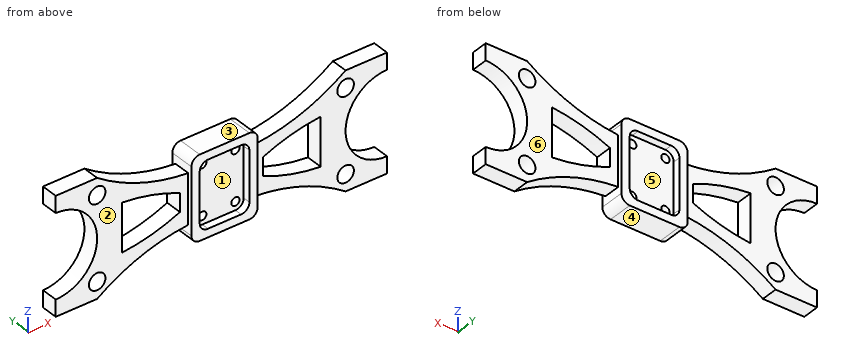
from build123d import *

# Parameters (mm, degrees)
SKETCH1_R             = 5
BOSS_EXTRUDE1_DEPTH   = 5
BOSS_EXTRUDE1_2_DEPTH = 5
SKETCH1_3_R           = 2.5
BOSS_EXTRUDE2_DEPTH   = 3
BOSS_EXTRUDE3_DEPTH   = 7.5


with BuildPart() as part:
    # Sketch1 → Boss-Extrude1 (new, symmetric)
    with BuildSketch(Plane(origin=(0, 0, 0), x_dir=(1, 0, 0), z_dir=(0, 1, 0))):
        with BuildLine():
            ThreePointArc((-75, -35), (-48.85448144, -21.27517604), (-20, -15))
            Line((-20, -15), (-20, 15))
            ThreePointArc((-20, 15), (-48.85448144, 21.27517604), (-75, 35))
            Line((-75, 35), (-100, 35))
            Line((-100, 35), (-100, 25))
            ThreePointArc((-100, 25), (-75, 0), (-100, -25))
            Line((-100, -25), (-100, -35))
            Line((-100, -35), (-75, -35))
        make_face()
        with Locations(Location((-75, -25, 0), (0, 0, 270))):
            Circle(SKETCH1_R, mode=Mode.SUBTRACT)
        with BuildLine():
            Line((-60, -14.5), (-60, 14.5))
            ThreePointArc((-60, 14.5), (-42.12787297, 11.447160671), (-25, 5.5))
            Line((-25, 5.5), (-25, -5.5))
            ThreePointArc((-25, -5.5), (-42.12787297, -11.447160671), (-60, -14.5))
        make_face(mode=Mode.SUBTRACT)
        with Locations(Location((-75, 25, 0), (0, 0, 270))):
            Circle(SKETCH1_R, mode=Mode.SUBTRACT)
    extrude(amount=BOSS_EXTRUDE1_DEPTH, both=True)



with BuildPart() as body_2:
    # Sketch1 → Boss-Extrude1 2 (new, symmetric)
    with BuildSketch(Plane(origin=(0, 0, 0), x_dir=(1, 0, 0), z_dir=(0, 1, 0))):
        with BuildLine():
            Line((20, 15), (20, -15))
            ThreePointArc((20, -15), (48.85448144, -21.27517604), (75, -35))
            Line((75, -35), (100, -35))
            Line((100, -35), (100, -25))
            ThreePointArc((100, -25), (75, 0), (100, 25))
            Line((100, 25), (100, 35))
            Line((100, 35), (75, 35))
            ThreePointArc((75, 35), (48.85448144, 21.27517604), (20, 15))
        make_face()
        with Locations(Location((75, -25, 0), (0, 0, 270))):
            Circle(SKETCH1_R, mode=Mode.SUBTRACT)
        with BuildLine():
            ThreePointArc((60, -14.5), (42.12787297, -11.447160671), (25, -5.5))
            Line((25, -5.5), (25, 5.5))
            ThreePointArc((25, 5.5), (42.12787297, 11.447160671), (60, 14.5))
            Line((60, 14.5), (60, -14.5))
        make_face(mode=Mode.SUBTRACT)
        with Locations(Location((75, 25, 0), (0, 0, 270))):
            Circle(SKETCH1_R, mode=Mode.SUBTRACT)
    extrude(amount=BOSS_EXTRUDE1_2_DEPTH, both=True)


with BuildPart() as body_3:
    # Sketch1<3> → Boss-Extrude2 (new, symmetric)
    with BuildSketch(Plane(origin=(0, 0, 0), x_dir=(1, 0, 0), z_dir=(0, 1, 0))):
        with BuildLine():
            Line((15, 15), (15, -15))
            ThreePointArc((15, -15), (13.535533906, -18.535533906), (10, -20))
            Line((10, -20), (-10, -20))
            ThreePointArc((-10, -20), (-13.535533906, -18.535533906), (-15, -15))
            Line((-15, -15), (-15, 15))
            ThreePointArc((-15, 15), (-13.535533906, 18.535533906), (-10, 20))
            Line((-10, 20), (10, 20))
            ThreePointArc((10, 20), (13.535533906, 18.535533906), (15, 15))
        make_face()
        with Locations(Location((10, 15, 0), (0, 0, 270))):
            Circle(SKETCH1_3_R, mode=Mode.SUBTRACT)
        with Locations(Location((-10, 15, 0), (0, 0, 270))):
            Circle(SKETCH1_3_R, mode=Mode.SUBTRACT)
        with Locations(Location((-10, -15, 0), (0, 0, 270))):
            Circle(SKETCH1_3_R, mode=Mode.SUBTRACT)
        with Locations(Location((10, -15, 0), (0, 0, 270))):
            Circle(SKETCH1_3_R, mode=Mode.SUBTRACT)
    extrude(amount=BOSS_EXTRUDE2_DEPTH, both=True)


with BuildPart() as part_1:
    add(part.part)

    add(body_2.part)  # Boss-Extrude3 merges body 2

    add(body_3.part)  # Boss-Extrude3 merges body 3
    # Sketch1<4> → Boss-Extrude3 (add, symmetric)
    with BuildSketch(Plane(origin=(0, 0, 0), x_dir=(1, 0, 0), z_dir=(0, 1, 0))):
        with BuildLine():
            ThreePointArc((-15, -25), (-18.535533906, -23.535533906), (-20, -20))
            Line((-20, -20), (-20, 20))
            ThreePointArc((-20, 20), (-18.535533906, 23.535533906), (-15, 25))
            Line((-15, 25), (15, 25))
            ThreePointArc((15, 25), (18.535533906, 23.535533906), (20, 20))
            Line((20, 20), (20, -20))
            ThreePointArc((20, -20), (18.535533906, -23.535533906), (15, -25))
            Line((15, -25), (-15, -25))
        make_face()
        with BuildLine():
            ThreePointArc((15, 15), (13.535533906, 18.535533906), (10, 20))
            Line((10, 20), (-10, 20))
            ThreePointArc((-10, 20), (-13.535533906, 18.535533906), (-15, 15))
            Line((-15, 15), (-15, -15))
            ThreePointArc((-15, -15), (-13.535533906, -18.535533906), (-10, -20))
            Line((-10, -20), (10, -20))
            ThreePointArc((10, -20), (13.535533906, -18.535533906), (15, -15))
            Line((15, -15), (15, 15))
        make_face(mode=Mode.SUBTRACT)
    extrude(amount=BOSS_EXTRUDE3_DEPTH, both=True)


solid = part_1.part
Could you check a few things on this model? Use its own coordinates, in mm. Face numbers are marked on the shaded views. A direction names the side the tool comes from. Give positions to 0.01 mm unless a question says otherwise; leave off trailing zeros. Loops run counter-clockwise (first coordinate to the right, second up) from the corner with the lowest first, then second, coordinate; pieces in that order, holes last. Notation, with made-up numbers: (8.25, 11.5) -> (21.25, 11.5) arc R30 cw to (21.25, 43.5) -> close; hole circle Ø3 at (17.25, 60). An arc over 180 degrees is marked (long way). Answer as CSV lines item,"result". Start each with the question number.
(1) If we section it at A-A on x = -86.5: Write out the boundary of the cut face in (y, z), then the cut area to 3 significant figures.
(2) If we section it at B-B on z = 2: Write out the boundary of the cut face in (x, y).
(3) I need wall thicknesses on probe 1 along X at (y, z) = (-2, -1); probe 2 along Z at (x, y) = (-9, -5.5); probe 3 along Y at (x, z) = (-89, 24.5). Which ranges of each line are inside material? Lowest first, please.
(4) Which directions (+Z, -Z, +X, -X, +Y, -Y) give clear straight access to the entire face, cutting with the end or side of a thin tool? Please do the marked faces 1, 2 and 3.
(5) If we section it at D-D on x = -2: Write out the boundary of the cut face in (y, z), then the cut area to 3 significant figures.
(6) I'm going to push flat-ended pins straight in: pin 1 Ø24 at (x, z) = (-2, -4) entering from +Y; pin 2 Ø9 at (x, z) = (75, 25) entering from -Y; pin 3 Ø5 at (y, z) = (-5, -0.5) entering from +X; pin 4 Ø3.5 at (x, y) = (1.5, 5.5) entering from -Z. Where does each tip first touch, or does it pass through?
(7) If we section it at C-C on y = 1: Count the separate pieces of the cut face and the enclosed holes in it, then the cut area to 3 significant figures.
(8) We'd pull the mould along Z, two halves only. Please class the marked faces 4, 5 and 6: released by +Z, released by -Z, zero draft, split by the parting line, or undercut.
Computed:
1,outline,"(-5, -35) -> (5, -35) -> (5, -21.04) -> (-5, -21.04) -> close; (-5, 21.04) -> (5, 21.04) -> (5, 35) -> (-5, 35) -> close"
1,area,"279 mm2"
2,outline,"(-75.08, -5) -> (-60, -5) -> (-60, 5) -> (-75.08, 5) -> close; (-25, -5) -> (-20, -5) -> (-20, -7.5) -> (-15, -7.5) -> (-15, -3) -> (15, -3) -> (15, -7.5) -> (20, -7.5) -> (20, -5) -> (25, -5) -> (25, 5) -> (20, 5) -> (20, 7.5) -> (15, 7.5) -> (15, 3) -> (-15, 3) -> (-15, 7.5) -> (-20, 7.5) -> (-20, 5) -> (-25, 5) -> close; (60, -5) -> (75.08, -5) -> (75.08, 5) -> (60, 5) -> close"
3,probe 1,"x = -75.02 to -60, -25 to 25, 60 to 75.02"
3,probe 2,"z = -25 to -20, 20 to 25"
3,probe 3,"y = -5 to 5"
4,face 1,"-Y"
4,face 2,"+Z, -Z, -X, -Y"
4,face 3,"+Z, +Y, -Y"
5,outline,"(-7.5, -25) -> (7.5, -25) -> (7.5, -20) -> (3, -20) -> (3, 20) -> (7.5, 20) -> (7.5, 25) -> (-7.5, 25) -> (-7.5, 20) -> (-3, 20) -> (-3, -20) -> (-7.5, -20) -> close"
5,area,"390 mm2"
6,pin 1,"stops at y = 3"
6,pin 2,"passes through"
6,pin 3,"stops at x = 75.18"
6,pin 4,"stops at z = -25"
7,separate pieces,"1"
7,enclosed holes,"10"
7,area,"6,460 mm2"
8,face 4,"released by -Z"
8,face 5,"undercut"
8,face 6,"zero draft"
